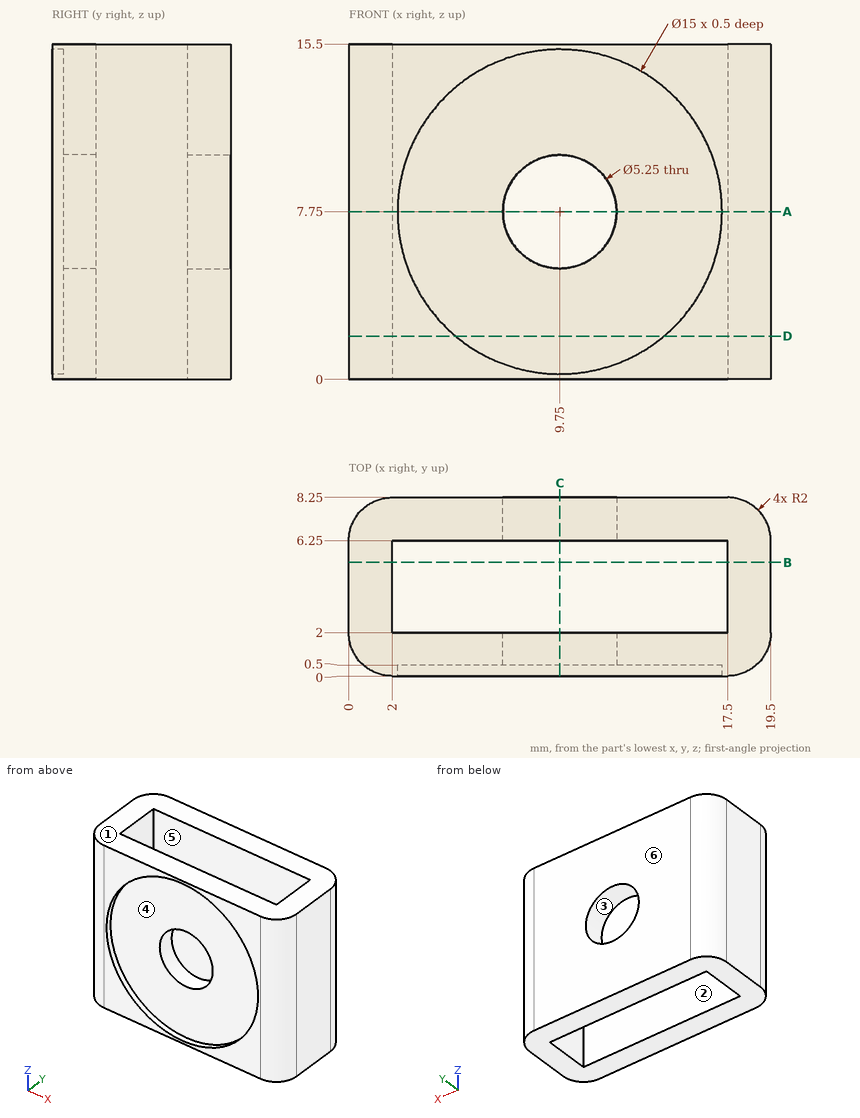
For this review, use the dimensioned drawing (mm, ordinates from the lowest corner) and the shaded views. A direction names the side the tool comes from. Round coordinates to 2 decimals unless told otherwise and drop trailing zeros. Order: outer loops, then holes, each group sorted by start corner. A loop starts at its lowest first (then second) coordinate and runs counter-clockwise, first axis right, second up. Notation, with made-up numbers: M 64,87 L 117,87 A20 ccw 117,91 Z; hole C -12,-0.5 d4. An arc over 180 degrees is marked long. Write each question's results on one line, items separated by ' | '. Start each with the question number.
1. Add section B-B (y = 5.25). State the section outline as (x, z) points.
2. To check wall thickness, follow L1, parallel to Y at x = 17.25, z = 5.5; L2, parallel to Z at x = 9.75, y = 7 (3 decimals); L3, parallel to Z at x = 9.75, y = 0.35. State the ranges of each line that lie inside material, in increasing order. Write a range as [from, to].
3. Add section A-A (z = 7.75). State the section outline as (x, y) points (3 decimals), then the cut area to 3 significant figures.
4. Clearance check with flat-ended pins moving along their axes: pin 1 Ø7 at (x, z) = (9.75, 7.75) entering from -Y; pin 2 Ø1.5 at (x, y) = (10, 3.5) entering from -Z. State where each tip first meets the part, or that it passes through.
5. Draft analysis for pull direction Z (two halves, no side actions). For the marked faces 1, 2 and 3, state which applies: pulls with the +Z half, pulls with the -Z half, needs draft (parallel to the pull), parting line crosses it, or undercut.
6. Tool access review of the marked faces 4, 5 and 6: name each direction out of +Z, -Z, +X, -X, +Y, -Y from which nothing blocks a thin tool from reaching the whole face with its end or side.
7. Add section D-D (z = 2). State the section outline as (x, y) points.
8. Add section C-C (x = 9.75). State the section outline as (y, z) points (3 decimals).
Output values:
1) outline: M 0,0 L 2,0 L 2,15.5 L 0,15.5 Z; M 17.5,0 L 19.5,0 L 19.5,15.5 L 17.5,15.5 Z
2) L1: [0, 2], [6.25, 8.25] | L2: [0, 5.125], [10.375, 15.5] | L3: [0, 0.25], [15.25, 15.5]
3) outline: M 0,2 A2 ccw 2,0 L 2.25,0 L 2.25,0.5 L 7.125,0.5 L 7.125,2 L 2,2 L 2,6.25 L 7.125,6.25 L 7.125,8.25 L 2,8.25 A2 ccw 0,6.25 Z; M 12.375,0.5 L 17.25,0.5 L 17.25,0 L 17.5,0 A2 ccw 19.5,2 L 19.5,6.25 A2 ccw 17.5,8.25 L 12.375,8.25 L 12.375,6.25 L 17.5,6.25 L 17.5,2 L 12.375,2 Z | area: 65.7 mm^2
4) pin 1: y = 0.5 | pin 2: through
5) face 1: pulls with the +Z half | face 2: needs draft | face 3: undercut
6) face 4: -Y | face 5: +Z, -Z | face 6: +Z, -Z, +X, -X, +Y
7) outline: M 0,2 A2 ccw 2,0 L 4.93,0 L 4.93,0.5 L 14.57,0.5 L 14.57,0 L 17.5,0 A2 ccw 19.5,2 L 19.5,6.25 A2 ccw 17.5,8.25 L 2,8.25 A2 ccw 0,6.25 Z; hole M 2,2 L 17.5,2 L 17.5,6.25 L 2,6.25 Z
8) outline: M 0,0 L 2,0 L 2,5.125 L 0.5,5.125 L 0.5,0.25 L 0,0.25 Z; M 0,15.25 L 0.5,15.25 L 0.5,10.375 L 2,10.375 L 2,15.5 L 0,15.5 Z; M 6.25,0 L 8.25,0 L 8.25,5.125 L 6.25,5.125 Z; M 6.25,10.375 L 8.25,10.375 L 8.25,15.5 L 6.25,15.5 Z
